Input: dimensioned drawing with shaded views. Units: mm. Origin: part minimum x, y, z. A direction names the side the tool comes from. Round coordinates to 2 decimals unless told otherwise and drop trailing zeros. Write each loop counter-clockwise with the first axis right and the second up, starting at its lowest first coordinate (ties: lowest second). Pieces come first, ordered by that corner, then holes. Notation, with made-up numbers: (50.25, -12) -> (61.25, -12) arc R21 ccw to (61.25, 20) -> close; hole circle Ø4 at (54.25, -8.75). An arc over 180 degrees is marked (long way). Use one line per item in the form item = value. Start each with the question number.
1. Draft query along Y for the marked faces 3, 4 and 5. Return one class per face: pulls with the +Y half, pulls with the -Y half, needs draft (parallel to the pull), parting line crosses it, or undercut.
2. Cut plane A-A, the plane x = 15. Return the cut outline in (y, z), plus the area to 3 significant figures.
3. Reachability of the marked faces 1 and 2 from +Z, -Z, +X, -X, +Y, -Y: full face, straight path, thin tool, end or side. Return the list, or none.
4. Line query: L1, parallel to Z at x = 1.75, y = 14; L2, parallel to Y at x = 15, z = 9; L3, parallel to X at y = 10.25, z = 18.5. Output: solid intervals per line, ascending.
5. Pin query (flat end, axial travel): pin 1 Ø1 at (x, z) = (18.5, 27.5) entering from +Y; pin 2 Ø5 at (y, z) = (4.5, 27) entering from +X; pin 3 Ø3 at (y, z) = (4.5, 17.5) entering from -X. Return the tip coordinate at first contact, or that it passes through.
6. Cut plane B-B, the plane z = 23. Return the cut outline in (x, y).
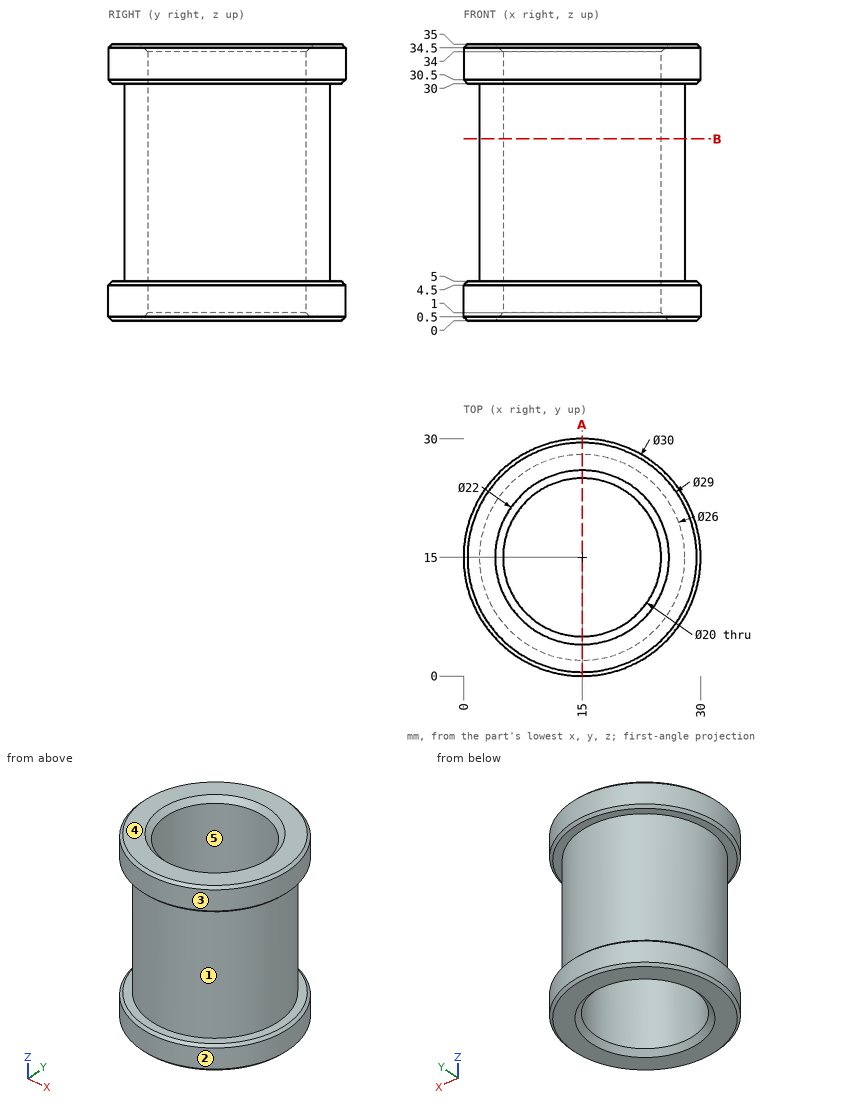
Outcome:
q1.face_3 = parting line crosses it
q1.face_4 = needs draft
q1.face_5 = undercut
q2.outline = (0, 0.5) -> (0.5, 0) -> (4, 0) -> (5, 1) -> (5, 34) -> (4, 35) -> (0.5, 35) -> (0, 34.5) -> (0, 30.5) -> (0.5, 30) -> (2, 30) -> (2, 5) -> (0.5, 5) -> (0, 4.5) -> close; (25, 1) -> (26, 0) -> (29.5, 0) -> (30, 0.5) -> (30, 4.5) -> (29.5, 5) -> (28, 5) -> (28, 30) -> (29.5, 30) -> (30, 30.5) -> (30, 34.5) -> (29.5, 35) -> (26, 35) -> (25, 34) -> close
q2.area = 247 mm^2
q3.face_1 = none
q3.face_2 = +Z, -Z
q4.L1 = 0 to 5, 30 to 35
q4.L2 = 2 to 5, 25 to 28
q4.L3 = 2.9 to 6.2, 23.8 to 27.1
q5.pin_1 = 27.65
q5.pin_2 = 25.25
q5.pin_3 = 5.62
q6.outline = circle Ø26 at (15, 15); hole circle Ø20 at (15, 15)
